Part model, mm, in its own coordinate system. Face numbers are marked on the shaded views. A direction names the side the tool comes from. Give positions to 0.01 mm unless a question says otherwise; leave off trailing zeros. Loops run counter-clockwise (first coordinate to the right, second up) from the corner with the lowest first, then second, coordinate; pieces in that order, holes last. Notation, with made-up numbers: M -14.5,67.25 L -3.5,67.25 A13 ccw -3.5,75.25 Z; hole C 88,23.5 d10. An arc over 180 degrees is marked long. Put each result on its own line as item: value. Start each with the question number.
```python
from build123d import *

# Parameters (mm, degrees)
SKETCH001_W     = 41.1
SKETCH001_H     = 23
PAD_DEPTH       = 13.2
SKETCH002_W     = 38.5
SKETCH002_H     = 20.6
POCKET_DEPTH    = 10.201
SKETCH_W        = 37.1
SKETCH_H        = 19
POCKET001_DEPTH = 2
SKETCH007_W     = 0.15
SKETCH007_H     = 3
SKETCH007_W_2   = 3
SKETCH007_H_2   = 0.15
PAD003_DEPTH    = 2


with BuildPart() as part:
    # Sketch001 (on DatumPlane) → Pad (new body)
    with BuildSketch(Plane.XY.offset(-3)):
        Rectangle(SKETCH001_W, SKETCH001_H)
    extrude(amount=PAD_DEPTH)

    # Sketch002 → Pocket (cut, through all)
    with BuildSketch(Plane.XY):
        Rectangle(SKETCH002_W, SKETCH002_H)
    extrude(amount=POCKET_DEPTH, mode=Mode.SUBTRACT)

    # Sketch → Pocket001 (cut)
    with BuildSketch(Plane.XY):
        Rectangle(SKETCH_W, SKETCH_H)
    extrude(amount=-POCKET001_DEPTH, mode=Mode.SUBTRACT)

    # Sketch007 (on DatumPlane) → Pad003 (join)
    with BuildSketch(Plane.XY.offset(1.6)):
        with Locations((-19.175, 0)):
            Rectangle(SKETCH007_W, SKETCH007_H)
        with Locations((0, 10.225)):
            Rectangle(SKETCH007_W_2, SKETCH007_H_2)
        with Locations((0, -10.225)):
            Rectangle(SKETCH007_W_2, SKETCH007_H_2)
        with Locations((19.175, 0)):
            Rectangle(SKETCH007_W, SKETCH007_H)
    extrude(amount=PAD003_DEPTH)


solid = part.part
```
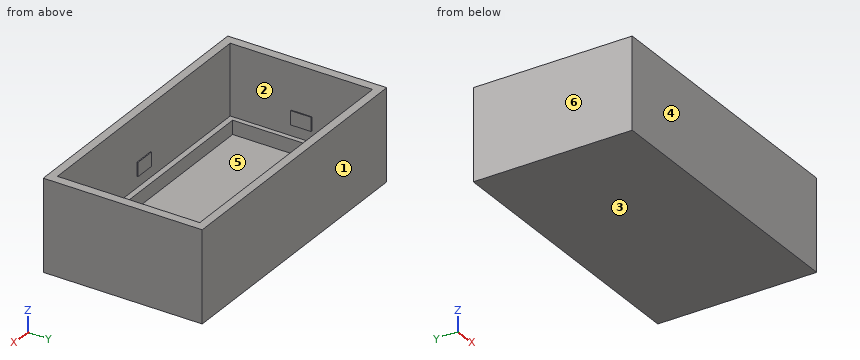
1) Pin check, flat tip, straight feed: pin 1 Ø6 at (x, y) = (-5, 4) entering from +Z. Stop position of the tip, or through.
2) Band-saw the part on C-C on x = 9. Give the cut face in (y, z).
3) Band-saw the part on D-D on z = -1.25. Give the cut face in (x, y).
4) Band-saw the part on A-A on z = 5.25. Give the cut face in (x, y).
5) Mould opens along Y. For the marked faces 1, 2, 3 and 4 say: +Y half, -Y half, draft (parallel to the pull), parting line (faces both ways), or undercut.
6) Band-saw the part on B-B on y = -0.5. Give the cut face in (x, z).
7) Wall check: L1, parallel to X at y = -10, z = 5; L2, parallel to Y at x = 16, z = 6.5; L3, parallel to Y at x = 7, z = -0.5. Give the ranges that are in metal, low to high.
8) Which spindle directions (+Z, -Z, +X, -X, +Y, -Y) get a long thin tool onto all of the face, cutting with end or side? Do the marked faces 5 and 6. Say none if no direction does.
Evaluation:
1. pin 1: z = -2
2. outline: M -11.5,-3 L 11.5,-3 L 11.5,10.2 L 10.3,10.2 L 10.3,0 L 9.5,0 L 9.5,-2 L -9.5,-2 L -9.5,0 L -10.3,0 L -10.3,10.2 L -11.5,10.2 Z
3. outline: M -20.55,-11.5 L 20.55,-11.5 L 20.55,11.5 L -20.55,11.5 Z; hole M -18.55,-9.5 L 18.55,-9.5 L 18.55,9.5 L -18.55,9.5 Z
4. outline: M -20.55,-11.5 L 20.55,-11.5 L 20.55,11.5 L -20.55,11.5 Z; hole M -19.25,-10.3 L 19.25,-10.3 L 19.25,10.3 L -19.25,10.3 Z
5. face 1: +Y half
5. face 2: undercut
5. face 3: draft
5. face 4: -Y half
6. outline: M -20.55,-3 L 20.55,-3 L 20.55,10.2 L 19.25,10.2 L 19.25,3.6 L 19.1,3.6 L 19.1,1.6 L 19.25,1.6 L 19.25,0 L 18.55,0 L 18.55,-2 L -18.55,-2 L -18.55,0 L -19.25,0 L -19.25,1.6 L -19.1,1.6 L -19.1,3.6 L -19.25,3.6 L -19.25,10.2 L -20.55,10.2 Z
7. L1: -20.55 to -19.25, 19.25 to 20.55
7. L2: -11.5 to -10.3, 10.3 to 11.5
7. L3: -11.5 to -9.5, 9.5 to 11.5
8. face 5: +Z
8. face 6: +Z, -Z, -X, +Y, -Y
